Autodesk Inventor part; units mm, degrees
ref_plane "YZ Plane" through (0, 0, 0) normal (1, 0, 0) x (0, 1, 0)
ref_plane "XZ Plane" through (0, 0, 0) normal (0, 1, 0) x (-1, 0, 0)
ref_plane "XY Plane" through (0, 0, 0) normal (0, 0, 1) x (1, 0, 0)
sketch "Sketch1" plane through (0, 0, 0) normal (0, 0, 1) x (1, 0, 0)
  line L0 (0, 0) -> (0, 5)
  line L1 (0, 5) -> (5, 5)
  line L2 (5, 5) -> (5, 0)
  line L3 (5, 0) -> (10, 0)
  line L4 (10, 0) -> (10, 5)
  line L5 (10, 5) -> (15, 5)
  line L6 (15, 5) -> (15, 0)
  line L7 (15, 0) -> (20, 0)
  line L8 (20, 0) -> (20, -5)
  line L9 (20, -5) -> (15, -5)
  line L10 (15, -5) -> (15, -10)
  line L11 (15, -10) -> (20, -10)
  line L12 (20, -10) -> (20, -15)
  line L13 (20, -15) -> (15, -15)
  line L14 (15, -15) -> (15, -20)
  line L15 (15, -20) -> (10, -20)
  line L16 (10, -20) -> (10, -15)
  line L17 (10, -15) -> (5, -15)
  line L18 (5, -15) -> (5, -20)
  line L19 (5, -20) -> (0, -20)
  line L20 (0, -20) -> (0, -15)
  line L21 (0, -15) -> (-5, -15)
  line L22 (-5, -15) -> (-5, -10)
  line L23 (-5, -10) -> (0, -10)
  line L24 (0, -10) -> (0, -5)
  line L25 (0, -5) -> (-5, -5)
  line L26 (-5, -5) -> (-5, 0)
  line L27 (-5, 0) -> (0, 0)
  dimension "d0" = 5
  dimension "d1" = 5
  dimension "d2" = 5
  dimension "d3" = 5
  dimension "d4" = 5
  dimension "d5" = 5
  dimension "d6" = 5
  dimension "d7" = 5
  dimension "d8" = 5
  dimension "d9" = 5
  dimension "d10" = 5
  dimension "d11" = 5
  dimension "d12" = 5
  dimension "d13" = 5
  dimension "d14" = 5
  dimension "d15" = 5
  dimension "d16" = 5
  dimension "d17" = 5
  dimension "d18" = 5
  dimension "d19" = 5
  dimension "d20" = 5
  dimension "d21" = 5
  dimension "d22" = 5
  dimension "d23" = 5
  dimension "d24" = 5
  dimension "d25" = 90
  dimension "d26" = 5
  dimension "d27" = 5
extrude "Extrusion1" add sketch "Sketch1" along normal blind 5
sketch "Sketch2" plane through (0, 0, 5) normal (0, 0, 1) x (1, 0, 0)
  line L0 (15, -10) -> (15, -5)
  line L1 (15, -7.5) -> (0, -7.5)
  line L2 (0, -10) -> (0, -5)
  circle A0 centre (7.5, -7.5) radius 1.75
  point P0 (0, 0)
  dimension "d30" = 3.5
extrude "Extrusion2" cut sketch "Sketch2" against normal blind 5
sketch "Sketch3" plane through (0, 0, 5) normal (0, 0, 1) x (1, 0, 0)
  circle A0 centre (7.5, -7.5) radius 1.75
  line L0 (7.5, -7.5) -> (10.5, -7.5)
  line L1 (10.5, -7.5) -> (9, -4.9019)
  line L2 (7.5, -7.5) -> (9, -4.9019)
  point P0 (0, 0)
  dimension "d33" = 3
  dimension "d34" = 3
  dimension "d35" = 60
extrude "Extrusion3" cut sketch "Sketch3" against normal blind 2.5 contours L0 L2 A0 | A0 L2 L1 L0 picked at (8.3623, -6.7236)
pattern_circular "Circular Pattern1" count 6 over 360 about axis through (7.5, -7.5, 5) along (0, 0, -1) of "Extrusion3"
sketch "Sketch4" plane through (-5, -15, 0) normal (0, -1, 0) x (1, 0, 0)
  line L0 (0, 5) -> (2.5, 5)
  line L1 (0, 5) -> (5, 5)
  line L2 (2.5, 5) -> (2.5, 2.5)
  circle A0 centre (2.5, 2.5) radius 1.75
  point P0 (5, 0)
  dimension "d41" = 2.5
  dimension "d42" = 2.5
  dimension "d43" = 3.5
extrude "Extrusion4" cut sketch "Sketch4" against normal through all
pattern_circular "Circular Pattern2" count 4 over 360 about axis through (7.5, -7.5, 5) along (0, 0, -1) of "Extrusion4"
properties part number "crossCenterMini"
The model under review builds one solid part; all positions refer to its coordinate system, in mm. A direction names the side the tool comes from. Coordinates: 2 decimals unless noted, no trailing zeros. Write each loop counter-clockwise with the first axis right and the second up, starting at its lowest first coordinate (ties: lowest second). Pieces come first, ordered by that corner, then holes. Notation, with made-up numbers: (18.25, 7.25) - (45.25, 7.25) arc R28 cw to (45.25, 29.25) - close; hole circle Ø6 at (54.25, 79.5). An arc over 180 degrees is marked (long way). Answer as a JSON object with one key per item and string values. Group by question number.
1. To check wall thickness, follow probe 1 along X at (y, z) = (-13.1, 2.5); probe 2 along Y at (x, z) = (10.25, 2.35); probe 3 along Y at (x, z) = (18.75, 0.25). State the ranges of each line that lie inside material, in increasing order.
2. Add section D-D (y = -13.75). Give the boundary of the cut face in (x, z), plus the area to 3 significant figures.
3. Add section A-A (x = -2.5). Give the boundary of the cut face in (y, z).
4. Add section B-B (y = 2.5). Give the boundary of the cut face in (x, z).
5. Machinability: for faces 1 (the face through (15, -7, 2)), 2 (the face through (5, 4, 1)), 3 (the face through (9, -6, 2.5)), 4 (the face through (10, -19, 1)), which of the approach directions +Z, -Z, +X, -X, +Y, -Y give a long, thin tool a straight path to every point of the face, cutting with its end or side? Answer none if there is none.
6. Add section C-C (x = 7.5). Give the boundary of the cut face in (y, z).
7. Mouldability with a two-part tool opening along X and no side actions: class faces 5 (the face through (18.89, -12.46, 1.44)), 6 (the face through (16, 0, 1)), 7 (the face through (-5, -13, 2)) as pulls with the +X half, pulls with the -X half, needs draft (parallel to the pull), parting line crosses it, or undercut.
8. Clearance check with flat-ended pins moving along their axes: pin 1 Ø2 at (x, z) = (7, 3.5) entering from -Y; pin 2 Ø1.2 at (x, z) = (7, 4) entering from +Y. State where each tip first meets the part, or that it passes through.
Findings:
{
 "1": {"probe 1": "-5 to -4.25, -0.75 to 15.75, 19.25 to 20", "probe 2": "-20 to -19.24, -15.76 to 0.76, 4.24 to 5", "probe 3": "-15 to -10, -5 to 0"},
 "2": {"outline": "(-5, 0) - (20, 0) - (20, 5) - (-5, 5) - close; hole circle Ø3.5 at (-2.5, 2.5); hole circle Ø3.5 at (17.5, 2.5)", "area": "106 mm²"},
 "3": {"outline": "(-15, 0) - (-10, 0) - (-10, 0.75) - (-15, 0.75) - close; (-15, 4.25) - (-10, 4.25) - (-10, 5) - (-15, 5) - close; (-5, 0) - (0, 0) - (0, 0.75) - (-5, 0.75) - close; (-5, 4.25) - (0, 4.25) - (0, 5) - (-5, 5) - close"},
 "4": {"outline": "(0, 0) - (5, 0) - (5, 0.75) - (0, 0.75) - close; (0, 4.25) - (5, 4.25) - (5, 5) - (0, 5) - close; (10, 0) - (15, 0) - (15, 0.75) - (10, 0.75) - close; (10, 4.25) - (15, 4.25) - (15, 5) - (10, 5) - close"},
 "5": {"face 1": "+Z, -Z, +X", "face 2": "+Z, -Z, +Y", "face 3": "+Z", "face 4": "+Z, -Z, -Y"},
 "6": {"outline": "(-15, 0) - (-9.25, 0) - (-9.25, 2.5) - (-10.1, 2.5) - (-10.1, 5) - (-15, 5) - close; (-5.75, 0) - (0, 0) - (0, 5) - (-4.9, 5) - (-4.9, 2.5) - (-5.75, 2.5) - close"},
 "7": {"face 5": "undercut", "face 6": "needs draft", "face 7": "pulls with the -X half"},
 "8": {"pin 1": "y = -15", "pin 2": "y = 0"}
}
